```python
from build123d import *

# Parameters (mm, degrees)
SKETCH_1_W          = 30
SKETCH_1_H          = 30
EXTRUDE_1_DEPTH     = 5
SKETCH_2_W          = 30
SKETCH_2_H          = 5
EXTRUDE_2_DEPTH     = 10
SKETCH_3_R          = 2.1
CUT_EXTRUDE_1_DEPTH = 5
EXTRUDE_3_DEPTH     = 20
SKETCH_5_W          = 35
SKETCH_5_H          = 5
EXTRUDE_4_DEPTH     = 10
SKETCH_6_W          = 35
SKETCH_6_H          = 5
EXTRUDE_5_DEPTH     = 10
SKETCH_7_R          = 2.1
CUT_EXTRUDE_2_DEPTH = 10
FILLET_1_R          = 6.17
FILLET_2_R          = 6.17
FILLET_3_R          = 6.17
FILLET_4_R          = 6.17


with BuildPart() as part:
    # 스케치1 → 보스-돌출1 (new body)
    with BuildSketch(Plane.XY):
        Rectangle(SKETCH_1_W, SKETCH_1_H)
    extrude(amount=EXTRUDE_1_DEPTH)

    # 스케치2 → 보스-돌출2 (add)
    with BuildSketch(Plane(origin=(0, 0, 0), x_dir=(-1, 0, 0), z_dir=(0, 0, -1))):
        with Locations((0, -12.5)):
            Rectangle(SKETCH_2_W, SKETCH_2_H)
    extrude(amount=EXTRUDE_2_DEPTH)

    # 스케치3 → 컷-돌출1 (cut)
    with BuildSketch(Plane(origin=(0, -10, 0), x_dir=(1, 0, 0), z_dir=(0, 1, 0))):
        with Locations((0, 5)):
            Circle(SKETCH_3_R)
    extrude(amount=-CUT_EXTRUDE_1_DEPTH, mode=Mode.SUBTRACT)

    # 스케치4 → 보스-돌출3 (add)
    with BuildSketch(Plane.XY.offset(5)):
        Polygon((10.2, -15), (15, -15), (15, 15), (-15, 15), (-15, -15), (-10.2, -15), (-10.2, 5.2), (10.2, 5.2), align=None)
    extrude(amount=EXTRUDE_3_DEPTH)

    # 스케치5 → 보스-돌출4 (add)
    with BuildSketch(Plane.ZY.offset(15)):
        with Locations((7.5, -12.5)):
            Rectangle(SKETCH_5_W, SKETCH_5_H)
    extrude(amount=EXTRUDE_4_DEPTH)

    # 스케치6 → 보스-돌출5 (add)
    with BuildSketch(Plane(origin=(15, 0, 0), x_dir=(0, 0, -1), z_dir=(1, 0, 0))):
        with Locations((-7.5, -12.5)):
            Rectangle(SKETCH_6_W, SKETCH_6_H)
    extrude(amount=EXTRUDE_5_DEPTH)

    # 스케치7 → 컷-돌출2 (cut)
    with BuildSketch(Plane(origin=(0, -10, 0), x_dir=(1, 0, 0), z_dir=(0, 1, 0))):
        with Locations((-20, -15)):
            Circle(SKETCH_7_R)
        with Locations((20, -15)):
            Circle(SKETCH_7_R)
    extrude(amount=-CUT_EXTRUDE_2_DEPTH, mode=Mode.SUBTRACT)

    # 필렛1
    fillet_1_edges = [part.edges().sort_by_distance(p)[0] for p in [
        (25, -12.5, 25),
    ]]
    fillet(fillet_1_edges, radius=FILLET_1_R)

    # 필렛2
    fillet_2_edges = [part.edges().sort_by_distance(p)[0] for p in [
        (25, -12.5, -10),
    ]]
    fillet(fillet_2_edges, radius=FILLET_2_R)

    # 필렛3
    fillet_3_edges = [part.edges().sort_by_distance(p)[0] for p in [
        (-25, -12.5, 25),
    ]]
    fillet(fillet_3_edges, radius=FILLET_3_R)

    # 필렛4
    fillet_4_edges = [part.edges().sort_by_distance(p)[0] for p in [
        (-25, -12.5, -10),
    ]]
    fillet(fillet_4_edges, radius=FILLET_4_R)


solid = part.part
```
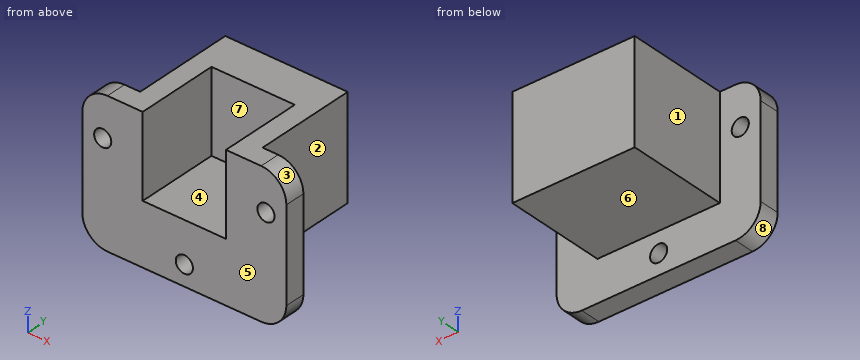
Can you work these out from the model? Positions are in its coordinate system, mm. Face numbers are marked on the shaded views. A direction names the side the tool comes from. Give positions to 0.01 mm unless a question says otherwise; leave off trailing zeros. Write each loop counter-clockwise with the first axis right and the second up, starting at its lowest first coordinate (ties: lowest second). Pieces come first, ordered by that corner, then holes. Notation, with made-up numbers: (34.5, 14.25) -> (60.5, 14.25) arc R12 cw to (60.5, 26.25) -> close; hole circle Ø1 at (-13.75, 61.5). An arc over 180 degrees is marked (long way). Write item = value, one per line.
(1) Suppose I cut it at C-C on y = -12.75. Write out the boundary of the cut face in (x, z), then the cut area to 3 significant figures.
Worked out:
outline = (-25, -3.83) arc R6.17 ccw to (-18.83, -10) -> (18.83, -10) arc R6.17 ccw to (25, -3.83) -> (25, 18.83) arc R6.17 ccw to (18.83, 25) -> (10.2, 25) -> (10.2, 5) -> (-10.2, 5) -> (-10.2, 25) -> (-18.83, 25) arc R6.17 ccw to (-25, 18.83) -> close; hole circle Ø4.2 at (-20, 15); hole circle Ø4.2 at (0, -5); hole circle Ø4.2 at (20, 15)
area = 1,270 mm^2
(2) I'm going to push flat-ended pins straight in: P1, Ø4, axis at y = 8.5, z = 7.5, coming from the -X side; P2, Ø16, axis at x = 1.5, y = -6.5, coming from the +Z side; P3, Ø1.5, axis at y = 6, z = -2.5, coming from the +X side; P4, Ø12.5, axis at y = -3, z = 17, coming from the +X side. Where does each tip first touch, or does it pass through?
Worked out:
P1 = -15
P2 = 5
P3 = through
P4 = 15
(3) Suppose I cut it at A-A on z = 15. Write out the boundary of the cut face in (x, y), then the cut area to 3 significant figures.
Worked out:
outline = (-25, -15) -> (-22.1, -15) -> (-22.1, -10) -> (-25, -10) -> close; (-17.9, -15) -> (-10.2, -15) -> (-10.2, 5.2) -> (10.2, 5.2) -> (10.2, -15) -> (17.9, -15) -> (17.9, -10) -> (15, -10) -> (15, 15) -> (-15, 15) -> (-15, -10) -> (-17.9, -10) -> close; (22.1, -15) -> (25, -15) -> (25, -10) -> (22.1, -10) -> close
area = 546 mm^2
(4) Thinking about a two-plate mould opening in X: for the marked faces 6, 7 and 8, which applies, released by +X, released by -X, zero draft, split by the parting line, or undercut?
Worked out:
face_6 = zero draft
face_7 = undercut
face_8 = released by -X
(5) For the marked faces 1, 2, 3, 4 and 5, which set-ups out of +Z, -Z, +X, -X, +Y, -Y let a thin tool reach every point of the face, with its end or its side?
Worked out:
face_1 = +Z, -Z, -X, +Y
face_2 = +Z, -Z, +X, +Y
face_3 = +Z, +X, +Y, -Y
face_4 = +Z, -Y
face_5 = +Z, -Z, +X, -X, -Y
(6) Suppose I cut it at B-B on x = 0. Write out the boundary of the cut face in (y, z).
Worked out:
outline = (-15, -10) -> (-10, -10) -> (-10, -7.1) -> (-15, -7.1) -> close; (-15, -2.9) -> (-10, -2.9) -> (-10, 0) -> (15, 0) -> (15, 25) -> (5.2, 25) -> (5.2, 5) -> (-15, 5) -> close
(7) I need wall thicknesses on probe 1 along X at (y, z) = (-12.65, 15); probe 2 along X at (y, z) = (-0.25, 6.5); probe 3 along Y at (x, z) = (-3, 16.5). Which ranges of each line are inside material? Lowest first, please. Write a range as from..to.
Worked out:
probe_1 = -25..-22.1, -17.9..-10.2, 10.2..17.9, 22.1..25
probe_2 = -15..-10.2, 10.2..15
probe_3 = 5.2..15
(8) Suppose I cut it at D-D on z = 6. Write out the boundary of the cut face in (x, y), then the cut area to 3 significant figures.
Worked out:
outline = (-25, -15) -> (-10.2, -15) -> (-10.2, 5.2) -> (10.2, 5.2) -> (10.2, -15) -> (25, -15) -> (25, -10) -> (15, -10) -> (15, 15) -> (-15, 15) -> (-15, -10) -> (-25, -10) -> close
area = 588 mm^2
